Source: CAD feature listing. Evaluate the final solid. Frame: model axes, mm. Face numbers are marked on the shaded views. A direction names the side the tool comes from. Round coordinates to 2 decimals unless told otherwise and drop trailing zeros. Write each loop counter-clockwise with the first axis right and the second up, starting at its lowest first coordinate (ties: lowest second). Pieces come first, ordered by that corner, then holes. Notation, with made-up numbers: M 17,-36 L 41,-36 A14 cw 41,-9 Z; hole C -31,77 d3. An arc over 180 degrees is marked long. Answer in a Markdown table with one row per item. Add a question column.
Item 1: Cut plane C-C on y = 6.5. Return loops of the section in (x, z), and give its area (3 significant figures).
Item 2: Cut plane B-B on x = 6.25. Return loops of the section in (y, z), and give its area (3 significant figures).
Item 3: Set-up query: the marked faces 1 and 2. Return all of +Z, -Z, +X, -X, +Y, -Y with unobstructed straight access to the full face (end or side cutting, diameter ignored); none if empty.
Item 4: Material intervals for probe 1 along Z at (x, y) = (-5, 4.5); probe 2 along Y at (x, z) = (3, 34); probe 3 along Z at (x, y) = (1.5, 1), sorted ascending.
Item 5: Cut plane A-A on z = 48.5. Return loops of the section in (x, y), and give its area (3 significant figures).
Item 6: Contact query for flat-ended pins moving along their axis: pin 1 (1.8 mm diameter, centred on x = 0.5, y = -1, fed in from +Z); pin 2 (4 mm diameter, centred on y = -3.5, z = 15.5, fed in from -X); pin 3 (2 mm diameter, centred on y = -2, z = 69.5, fed in from +X); pin 4 (1 mm diameter, centred on x = -4.5, z = 90, fed in from -Y). Output: stop coordinate, or through.
from build123d import *

# Parameters (mm, degrees)
F0_R     = 8.5
F1_DEPTH = 4
F2_R     = 5
F3_DEPTH = 100
F7_DEPTH = 5


with BuildPart() as f1:
    # F0 (on Top) → F1 (new body)
    with BuildSketch(Plane.XY):
        Circle(F0_R)
    extrude(amount=F1_DEPTH)

    # F2 (on Top) → F3 (join)
    with BuildSketch(Plane.XY):
        Circle(F2_R)
    extrude(amount=F3_DEPTH)

    # F4 (on Right) → F5 (revolve)
    with BuildSketch(Plane.YZ):
        with BuildLine():
            Line((3, 102), (0, 102))
            Line((0, 102), (0, 100))
            Line((0, 100), (5, 100))
            ThreePointArc((5, 100), (3.585786, 100.585786), (3, 102))
        make_face()
    revolve(axis=Axis((0, 0, 101), (0, 0, -1)))

    # F6 (on face) → F7 (join)
    with BuildSketch(Plane.XY.offset(102)):
        Polygon((0.087017, -0.996207), (0.906249, -0.422744), (0.819232, 0.573463), (-0.087017, 0.996207), (-0.906249, 0.422744), (-0.819232, -0.573463), align=None)
    extrude(amount=F7_DEPTH)


solid = f1.part
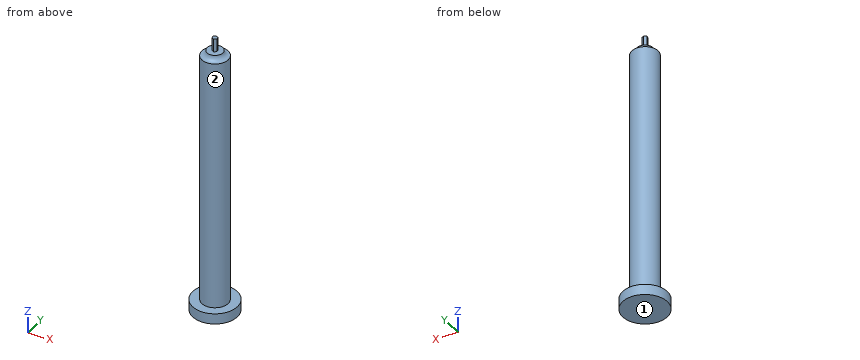
Results below:
| question | item | result |
|---|---|---|
| 1 | outline | M -5.48,0 L 5.48,0 L 5.48,4 L -5.48,4 Z |
| 1 | area | 43.8 mm2 |
| 2 | outline | M -5.76,0 L 5.76,0 L 5.76,4 L -5.76,4 Z |
| 2 | area | 46.1 mm2 |
| 3 | face 1 | -Z, +X, -X, +Y, -Y |
| 3 | face 2 | +Z |
| 4 | probe 1 | 0 to 4 |
| 4 | probe 2 | -4 to 4 |
| 4 | probe 3 | 0 to 102 |
| 5 | outline | C 0,0 d10 |
| 5 | area | 78.5 mm2 |
| 6 | pin 1 | z = 107 |
| 6 | pin 2 | x = -4.77 |
| 6 | pin 3 | x = 4.9 |
| 6 | pin 4 | y = -3 |
